Read the model definition and answer for the solid it produces. Units are mm, in the model's axes. Give positions to 0.01 mm unless a question says otherwise; leave off trailing zeros. Order: outer loops, then holes, each group sorted by start corner. A loop starts at its lowest first (then second) coordinate and runs counter-clockwise, first axis right, second up. Notation, with made-up numbers: (27.25, -37) - (74.25, -37) arc R22 ccw to (74.25, -3) - close; hole circle Ø10 at (11, 77.5). An arc over 180 degrees is marked (long way). Write each question's results on one line, items separated by ' | '. Start each with the question number.
Q1. Find section A-A on x = 66.5. Give the vertices of the cut face in (y, z), and give its area (3 significant figures).
Q2. Find the intervals of material crossed by line 1 along X through (y, z) = (1.35, -23.5); line 2 along X through (y, z) = (2.2, 20); line 3 along Z through (x, y) = (-69, 1.7), in increasing order. Write a range as from..to.
Q3. Flat-ended cylindrical pins translate along their axes: P1, Ø0.9, axis at y = 1, z = -26.5, coming from the -X side; P2, Ø1.5, axis at x = -128, y = 2, coming from the -Z side; P3, Ø1.5, axis at y = 1, z = -20.5, coming from the -X side. Find the tip coordinate at first contact, or state that the pin passes through.
from build123d import *

# Parameters (mm, degrees)
SKETCH2_W           = 260
SKETCH2_H           = 56
BOSS_EXTRUDE1_DEPTH = 3
SKETCH4_W           = 3
SKETCH4_H           = 15
CUT_EXTRUDE1_DEPTH  = 134.015036744


with BuildPart() as part:
    # Sketch2 → Boss-Extrude1 (new body)
    with BuildSketch(Plane(origin=(0, 0, 0), x_dir=(1, 0, 0), z_dir=(0, 1, 0))):
        Rectangle(SKETCH2_W, SKETCH2_H)
    extrude(amount=BOSS_EXTRUDE1_DEPTH)

    # Sketch4 → Cut-Extrude1 (cut, through all)
    with BuildSketch(Plane(origin=(0, 3, 0), x_dir=(1, 0, 0), z_dir=(0, 1, 0))):
        with Locations((-128.5, 0)):
            Rectangle(SKETCH4_W, SKETCH4_H)
        Polygon((-50, 25), (-50, 20.5), (-48.5, 20.5), (-48.5, 18), (-54.5, 18), (-54.5, 20.5), (-53, 20.5), (-53, 25), (-100, 25), (-100, 28), (-5, 28), (-5, 25), align=None)
        Polygon((-130, 28), (-130, 17.5), (-127, 17.5), (-127, 25), (-110, 25), (-110, 28), align=None)
        Polygon((110, 28), (130, 28), (130, 17.5), (127, 17.5), (127, 25), (110, 25), align=None)
        Polygon((5, 28), (5, 25), (50, 25), (50, 20.5), (48.5, 20.5), (48.5, 18), (54.5, 18), (54.5, 20.5), (53, 20.5), (53, 25), (100, 25), (100, 28), align=None)
        with Locations((128.5, 0)):
            Rectangle(SKETCH4_W, SKETCH4_H)
        Polygon((50, -25), (50, -20.5), (48.5, -20.5), (48.5, -18), (54.5, -18), (54.5, -20.5), (53, -20.5), (53, -25), (100, -25), (100, -28), (5, -28), (5, -25), align=None)
        Polygon((130, -28), (130, -17.5), (127, -17.5), (127, -25), (110, -25), (110, -28), align=None)
        Polygon((-110, -28), (-130, -28), (-130, -17.5), (-127, -17.5), (-127, -25), (-110, -25), align=None)
        Polygon((-5, -28), (-5, -25), (-50, -25), (-50, -20.5), (-48.5, -20.5), (-48.5, -18), (-54.5, -18), (-54.5, -20.5), (-53, -20.5), (-53, -25), (-100, -25), (-100, -28), align=None)
    extrude(amount=-CUT_EXTRUDE1_DEPTH, mode=Mode.SUBTRACT)


solid = part.part
Working result:
1) outline: (0, -25) - (3, -25) - (3, 25) - (0, 25) - close | area: 150 mm²
2) line 1: -127..-53, -50..50, 53..127 | line 2: -127..-54.5, -48.5..48.5, 54.5..127 | line 3: -25..25
3) P1: x = -110 | P2: z = -17.5 | P3: x = -127
